The model under review builds one solid part; all positions refer to its coordinate system, in mm. A direction names the side the tool comes from. Round coordinates to 2 decimals unless told otherwise and drop trailing zeros. Order: outer loops, then holes, each group sorted by start corner. A loop starts at its lowest first (then second) coordinate and runs counter-clockwise, first axis right, second up.
```python
from build123d import *

# Parameters (mm, degrees)
SKETCH1_W                 = 18
SKETCH1_H                 = 18
BOSS_EXTRUDE1_DEPTH       = 72
SKETCH2_R                 = 5
CUT_EXTRUDE1_DEPTH        = 19
M6X1_0_TAPPED_HOLE1_D     = 5
M6X1_0_TAPPED_HOLE1_DEPTH = 29
M6X1_0_TAPPED_HOLE1_TIP   = 1.502151548
SKETCH6_R                 = 7.5
CUT_EXTRUDE2_DEPTH        = 6


with BuildPart() as part:
    # Sketch1 → Boss-Extrude1 (new body)
    with BuildSketch(Plane(origin=(0, 0, 0), x_dir=(1, 0, 0), z_dir=(0, 1, 0))):
        with Locations((-33.958762887, 4.268041237)):
            Rectangle(SKETCH1_W, SKETCH1_H)
    extrude(amount=BOSS_EXTRUDE1_DEPTH)

    # Sketch2 → Cut-Extrude1 (cut, through all)
    with BuildSketch(Plane.XY.offset(4.731958763)):
        with Locations((-33.958762887, 57.2)):
            Circle(SKETCH2_R)
    extrude(amount=-CUT_EXTRUDE1_DEPTH, mode=Mode.SUBTRACT)

    # M6x1.0 Tapped Hole1
    with Locations(Plane(origin=(0, 0, 0), x_dir=(-1, 0, 0), z_dir=(0, -1, 0))):
        with Locations((33.958762887, 4.268041237)):
            Hole(M6X1_0_TAPPED_HOLE1_D / 2, depth=M6X1_0_TAPPED_HOLE1_DEPTH)
            with Locations((0, 0, -(M6X1_0_TAPPED_HOLE1_DEPTH + M6X1_0_TAPPED_HOLE1_TIP / 2))):  # 118° drill point
                Cone(0, M6X1_0_TAPPED_HOLE1_D / 2, M6X1_0_TAPPED_HOLE1_TIP, mode=Mode.SUBTRACT)

    # Sketch6 → Cut-Extrude2 (cut)
    with BuildSketch(Plane.XY.offset(4.731958763)):
        with Locations((-33.958762887, 57.2)):
            Circle(SKETCH6_R)
    extrude(amount=-CUT_EXTRUDE2_DEPTH, mode=Mode.SUBTRACT)


solid = part.part
```
(1) To check wall thickness, follow probe 1 along Y at (x, z) = (-34, -11.25); probe 2 along Y at (x, z) = (-31, -1.5); probe 3 along X at (y, z) = (15.5, -5). State the ranges of each line that lie inside material, in increasing order.
Data:
probe 1: y = 0 to 52.2, 62.2 to 72
probe 2: y = 0 to 53.17, 61.23 to 72
probe 3: x = -42.96 to -36.35, -31.57 to -24.96
(2) Consider section A-A (y = 57.2). Write out the cut boundary in (x, z).
Data:
outline: (-42.96, -13.27) - (-38.96, -13.27) - (-38.96, -1.27) - (-41.46, -1.27) - (-41.46, 4.73) - (-42.96, 4.73) - close; (-28.96, -13.27) - (-24.96, -13.27) - (-24.96, 4.73) - (-26.46, 4.73) - (-26.46, -1.27) - (-28.96, -1.27) - close
(3) Consider section B-B (z = 2.75). Write out the cut boundary in (x, y).
Data:
outline: (-42.96, 0) - (-24.96, 0) - (-24.96, 72) - (-42.96, 72) - close; hole circle Ø15 at (-33.96, 57.2)
(4) Consider section C-C (x = -30). Write out the cut boundary in (y, z).
Data:
outline: (0, -13.27) - (54.15, -13.27) - (54.15, -1.27) - (50.83, -1.27) - (50.83, 4.73) - (0, 4.73) - close; (60.25, -13.27) - (72, -13.27) - (72, 4.73) - (63.57, 4.73) - (63.57, -1.27) - (60.25, -1.27) - close
(5) Insertion check: pin 1 (6 mm diameter, centred on x = -33.96, y = 57.2, fed in from +Z). The pin has a flat end and moves straight along its axis. Give the tip position at first contact, or say it passes through.
Data:
pin 1: passes through
(6) Consider section D-D (y = 25.5). Write out the cut boundary in (x, z).
Data:
outline: (-42.96, -13.27) - (-24.96, -13.27) - (-24.96, 4.73) - (-42.96, 4.73) - close; hole circle Ø5 at (-33.96, -4.27)
(7) Draft analysis for pull direction Y (two halves, no side actions). For faces 3 (the flat face through (-34, 72, -4)), 4 (the cylindrical face through (-31.65, 14.7, -3.31)), 5 (the cylindrical face through (-35.585, 49.878, 1.774)), state which applies: pulls with the +Y half, pulls with the -Y half, needs draft (parallel to the pull), parting line crosses it, or undercut.
Data:
face 3: pulls with the +Y half
face 4: needs draft
face 5: undercut
(8) For faces 1 (the flat face through (-32, 52, -1.268)), 2 (the conical face through (-33.86, 30.24, -3.84)), list the 3-axis set-ups (+Z, -Z, +X, -X, +Y, -Y) from which the entire face can be reached by the end or side of a thin tool; tool diameter is ignored.
Data:
face 1: +Z
face 2: -Y
